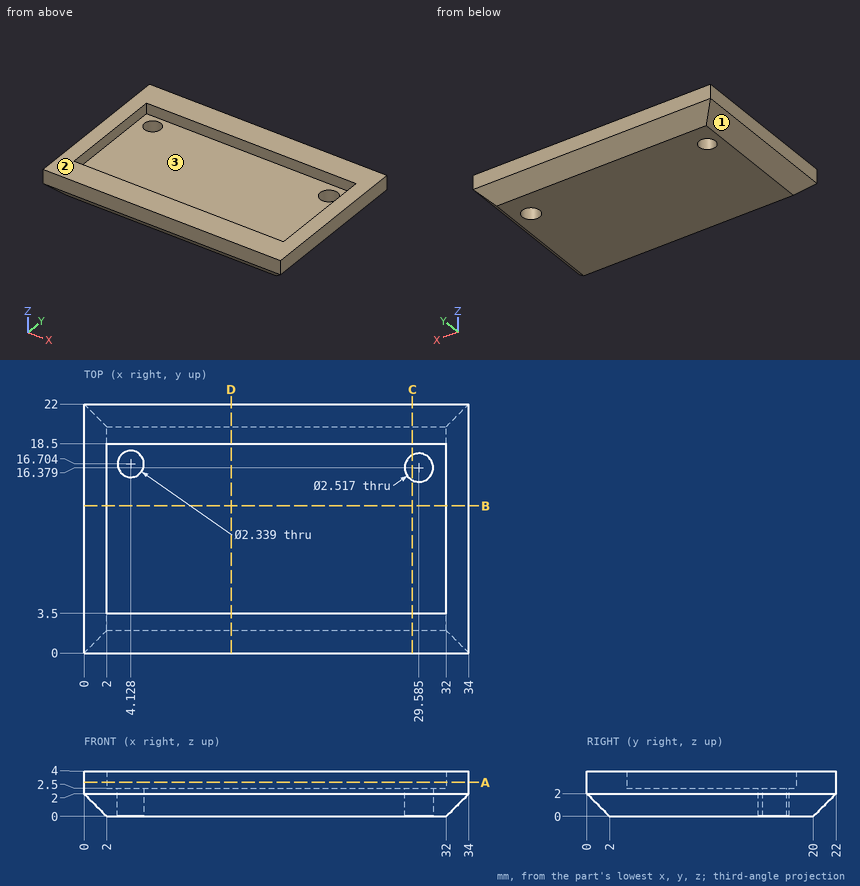
The drawing under review shows one solid part. Ordinate dimensions are in mm from its lowest x, y, z. Give positions to 0.01 mm unless a question says otherwise; leave off trailing zeros. Order: outer loops, then holes, each group sorted by start corner. A loop starts at its lowest first (then second) coordinate and runs counter-clockwise, first axis right, second up. Notation, with made-up numbers: (53, 50) - (63, 50) arc R11 cw to (63, 64) - close; hole circle Ø7 at (49.5, 17). An arc over 180 degrees is marked (long way). Answer as a JSON object with one key per item and string values. Group by question number.
Item 1: Draft analysis for pull direction X (two halves, no side actions). For the marked faces 1, 2 and 3, state which applies: pulls with the +X half, pulls with the -X half, needs draft (parallel to the pull), parting line crosses it, or undercut.
Item 2: Take a section at B-B on y = 13. Give the boundary of the cut face in (x, z).
Item 3: Clearance check with flat-ended pins moving along their axes: pin 1 Ø1.5 at (y, z) = (11, 0.5) entering from -X; pin 2 Ø8 at (x, y) = (27.5, 14) entering from +Z. State where each tip first meets the part, or that it passes through.
Item 4: Take a section at C-C on x = 29. Give the boundary of the cut face in (y, z) (1 decimal).
Item 5: Take a section at D-D on x = 13. Give the boundary of the cut face in (y, z).
Item 6: Take a section at A-A on z = 3. Give the boundary of the cut face in (x, y), and give its area (3 significant figures).
Item 7: Wall thickness on line 1 along Y through (x, z) = (30.5, 3.1); line 2 along X through (y, z) = (10, 3.45); line 3 along Z through (x, y) = (10, 7.75): over which ranges is each line inside the solid? List them lowest first.
Reported:
{
 "1": {"face 1": "pulls with the -X half", "face 2": "needs draft", "face 3": "undercut"},
 "2": {"outline": "(0, 2) - (2, 0) - (32, 0) - (34, 2) - (34, 4) - (32, 4) - (32, 2.5) - (2, 2.5) - (2, 4) - (0, 4) - close"},
 "3": {"pin 1": "x = 0.75", "pin 2": "z = 2.5"},
 "4": {"outline": "(0, 2) - (2, 0) - (15.3, 0) - (15.3, 2.5) - (3.5, 2.5) - (3.5, 4) - (0, 4) - close; (17.5, 0) - (20, 0) - (22, 2) - (22, 4) - (18.5, 4) - (18.5, 2.5) - (17.5, 2.5) - close"},
 "5": {"outline": "(0, 2) - (2, 0) - (20, 0) - (22, 2) - (22, 4) - (18.5, 4) - (18.5, 2.5) - (3.5, 2.5) - (3.5, 4) - (0, 4) - close"},
 "6": {"outline": "(0, 0) - (34, 0) - (34, 22) - (0, 22) - close; hole (2, 3.5) - (32, 3.5) - (32, 18.5) - (2, 18.5) - close", "area": "298 mm^2"},
 "7": {"line 1": "0 to 3.5, 18.5 to 22", "line 2": "0 to 2, 32 to 34", "line 3": "0 to 2.5"}
}
